Part model, mm, in its own coordinate system. A direction names the side the tool comes from. Give positions to 0.01 mm unless a question says otherwise; leave off trailing zeros. Order: outer loops, then holes, each group sorted by start corner. A loop starts at its lowest first (then second) coordinate and runs counter-clockwise, first axis right, second up. Notation, with made-up numbers: (69, 29) - (104, 29) arc R22 ccw to (104, 58) - close; hole circle Ø10 at (31, 31.5). An arc over 180 degrees is marked (long way). One line per item, written item: value.
Autodesk Inventor part; units mm, degrees
ref_plane "Work Plane1" through (0, 9.525, 0) normal (0, 1, 0) x (-1, 0, 0)
ref_plane "YZ Plane" through (0, 0, 0) normal (1, 0, 0) x (0, 1, 0)
ref_plane "XY Plane" through (0, 0, 0) normal (0, 0, 1) x (1, 0, 0)
sketch "Sketch1" plane through (0, 0, 0) normal (0, 0, 1) x (1, 0, 0)
  line L0 (2.7496, 4.7625) -> (5.4993, 0)
  line L1 (5.4993, 0) -> (2.7496, -4.7625)
  line L2 (2.7496, -4.7625) -> (-2.7496, -4.7625)
  line L3 (-2.7496, -4.7625) -> (-5.4993, 0)
  line L4 (-5.4993, 0) -> (-2.7496, 4.7625)
  line L5 (-2.7496, 4.7625) -> (2.7496, 4.7625)
  circle A0 centre (0, 0) radius 9.525
  circle A1 centre (0, 0) radius 5.4993 construction
  dimension "d0" = 9.525
  dimension "d2" = 19.05
  dimension "d3" = 4.0257
extrude "Extrusion1" add sketch "Sketch1" against normal blind 19.05
thicken "Thicken Hex" operation add thickness 0.127 both sides no extend neighbours yes toward (-0.8660254, 0.5, 0) faces at (-4.5827, 1.5875, -6.35) (-3.6662, -3.175, -6.35) (0.9165, -4.7625, -6.35) (-0.9165, 4.7625, -6.35) (3.6662, 3.175, -6.35) (4.5827, -1.5875, -6.35)
ref_plane "Work Plane1" through (0, 9.525, 0) normal (0, 1, 0) x (-1, 0, 0)
sketch "Sketch3" plane through (0, 9.525, 0) normal (0, 1, 0) x (-1, 0, 0)
  line L0 (0, 0) -> (0, -19.05) construction
  line L1 (-9.525, -19.05) -> (9.525, -19.05) construction
  point P0 (0, -9.525)
hole "Hole1" at (0, 9.525, -9.525) direction (0, -1, 0) diameter 3.81 end through all
equation "\"d0\" = hexSize"
equation "\"d2\" = exteriorDiameter"
equation "\"d4\" = length"
equation "\"d6\" = printSpacing"
equation "\"d7\" = printSpacing"
equation "\"hexSize\" = 9.525"
equation "\"exteriorDiameter\" = 19.05"
equation "\"length\" = 19.05"
equation "\"printSpacing\" = 0.127"
properties part number "3_8x3_4x3_4-hexBearing" material "PC/ABS Plastic"
1) Two-plate mould, pull along X, no slides. Class faces 3 (the face through (4.215, 2.479, -9.392)), 4 (the face through (4, -4, 0)), 5 (the face through (-2.06, -9.3, -9.39)): pulls with the +X half, pulls with the -X half, needs draft (parallel to the pull), parting line crosses it, or undercut.
Answer:
face 3: undercut
face 4: needs draft
face 5: parting line crosses it
2) Slice it at A-A on x = 0. Count the separate pieces of the cut face and the enclosed holes in it, then the cut area to 3 significant figures.
Answer:
separate pieces: 4
enclosed holes: 0
area: 141 mm2
3) Slice it at D-D on y = 8. Write the cut outline in (x, z) (3 decimals).
Answer:
outline: (-5.17, -19.05) - (5.17, -19.05) - (5.17, 0) - (-5.17, 0) - close; hole circle Ø3.81 at (0, -9.525)
4) Wall check: line 1 along Z through (x, y) = (0, 5.95); line 2 along Y through (x, z) = (5, -16.5); line 3 along Y through (x, z) = (4, -5.5). Give the ranges that are in metal, low to high. Write a range as [from, to].
Answer:
line 1: z = [-19.05, -11.43], [-7.62, 0]
line 2: y = [-8.11, -1.12], [1.12, 8.11]
line 3: y = [-8.64, -2.85], [2.85, 8.64]
5) Drop flat-ended pins along their axis: P1, Ø1.5, axis at y = -2, z = -7.5, coming from the -X side; P2, Ø1.5, axis at x = -3, y = -2, coming from the -Z side; P3, Ø1, axis at y = 3, z = -11.5, coming from the +X side; P4, Ø3, axis at x = -6, z = -16.5, coming from the +Y side (3 decimals). Give the stop position or say it passes through.
Answer:
P1: stops at x = -9.44
P2: passes through
P3: stops at x = 9.19
P4: stops at y = 8.395
6) Which spindle directions (+Z, -Z, +X, -X, +Y, -Y) get a long thin tool onto all of the face, cutting with end or side? Do faces 1 (the face through (-0.572, 7.175, -7.708)), 2 (the face through (4.254, -2.411, -9.392)). Say none if no direction does.
Answer:
face 1: +Y, -Y
face 2: +Z, -Z
7) Slice it at C-C on x = -4.5. Write the cut outline in (y, z), then the cut area to 3 significant figures.
Answer:
outline: (-8.39, -19.05) - (-1.98, -19.05) - (-1.98, 0) - (-8.39, 0) - close; (1.98, -19.05) - (8.39, -19.05) - (8.39, 0) - (1.98, 0) - close
area: 244 mm2
